The model under review builds one solid part; all positions refer to its coordinate system, in mm. Face numbers are marked on the shaded views. A direction names the side the tool comes from. Round coordinates to 2 decimals unless told otherwise and drop trailing zeros. Order: outer loops, then holes, each group sorted by start corner. A loop starts at its lowest first (then second) coordinate and runs counter-clockwise, first axis right, second up.
1) Machinability: for the marked faces 1 and 2, which of the approach directions +Z, -Z, +X, -X, +Y, -Y give a long, thin tool a straight path to every point of the face, cutting with its end or side? Answer none if there is none.
2) Consider section D-D (z = 58.5). Give the boundary of the cut face in (x, y).
3) Consider section A-A (z = 81.5). Give the boundary of the cut face in (x, y), then the cut area to 3 significant figures.
4) Clearance check with flat-ended pins moving along their axes: P1, Ø4, axis at x = -17.5, y = 30, coming from the -Z side; P2, Ø4, axis at x = -62, z = 31, coming from the +Y side; P3, Ø6, axis at x = 20, y = 43.5, coming from the +Z side; P4, Ø3, axis at x = 71, z = 31, coming from the -Y side. State where each tip first meets the part, or that it passes through.
5) To check wall thickness, follow L1, parallel to X at y = 2.5, z = 32; L2, parallel to Y at x = -85, z = 45.5; L3, parallel to X at y = -57.5, z = 76. State the ranges of each line that lie inside material, in increasing order.
6) Consider section C-C (y = 27.5). Give the boundary of the cut face in (x, z).
7) Consider section B-B (x = 53). Give the boundary of the cut face in (y, z), then the cut area to 3 significant figures.
from build123d import *
from build123d import SkipClean  # not in build123d's __all__

# Parameters (mm, degrees)
F1_DEPTH = 100
F3_DEPTH = 20
F4_DEPTH = 50


with BuildPart() as f1:
    # F0 (on Top) → F1 (new body)
    with BuildSketch(Plane.XY):
        with BuildLine():
            Line((-100, -50), (0, -50))
            Line((0, -50), (0, 0))
            Line((0, 0), (-75.3427499533, 0))
            ThreePointArc((-75.3427499533, 0), (-85.3427499533, -10), (-95.3427499533, 0))
            Line((-95.3427499533, 0), (-100, 0))
            Line((-100, 0), (-100, -50))
        make_face()
    extrude(amount=F1_DEPTH)

    # F2 (on face) → F3 (join)
    with BuildSketch(Plane.XZ.offset(50)):
        with BuildLine():
            ThreePointArc((0, 70), (-21.2132034356, 78.7867965644), (-30, 100))
            Line((-30, 100), (-60, 100))
            ThreePointArc((-60, 100), (-42.4264068712, 57.5735931288), (0, 40))
            Line((0, 40), (0, 70))
        make_face()
    extrude(amount=F3_DEPTH)

    # F4 (cut, through all): a face of the model
    f4_faces = [f1.faces().sort_by_distance(p)[0] for p in [
        (-12.7323954474, -50, 87.2676045526),
    ]]
    extrude(f4_faces, amount=-F4_DEPTH, mode=Mode.SUBTRACT)

    # F5: F1 across plane


with BuildPart() as f1_1:
    add(f1.part, clean=False)
    with SkipClean():  # cleaning this boolean's faces spoils the solid; the shape is the same uncleaned
        add(f1.part.mirror(Plane.XZ), clean=False)

    # F6: F1 across face


with BuildPart() as f1_2:
    add(f1_1.part, clean=False)
    add(f1_1.part.mirror(Plane(origin=(0, -30.1219512195, 37.9268292683), x_dir=(0, 1, 0), z_dir=(1, 0, 0))), clean=False)


solid = f1_2.part
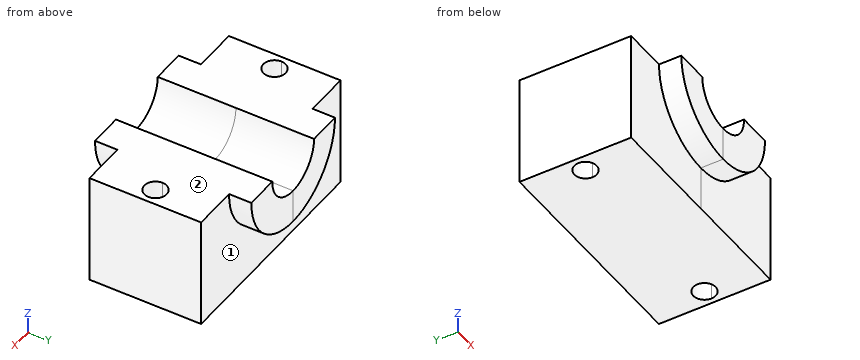
Answer below:
1. face 1: -Z, +Y
1. face 2: +Z, +X, -X, +Y, -Y
2. outline: (-100, -50) - (-43.33, -50) - (-43.33, -70) - (43.33, -70) - (43.33, -50) - (100, -50) - (100, 50) - (43.33, 50) - (43.33, 70) - (-43.33, 70) - (-43.33, 50) - (-100, 50) - close; hole circle Ø20 at (-85.34, 0); hole circle Ø20 at (85.34, 0)
3. outline: (-100, -50) - (-57.08, -50) - (-57.08, -70) - (-23.62, -70) - (-23.62, 70) - (-57.08, 70) - (-57.08, 50) - (-100, 50) - close; (23.62, -70) - (57.08, -70) - (57.08, -50) - (100, -50) - (100, 50) - (57.08, 50) - (57.08, 70) - (23.62, 70) - close; hole circle Ø20 at (-85.34, 0); hole circle Ø20 at (85.34, 0)
3. area: 17,300 mm2
4. P1: stops at z = 0
4. P2: stops at y = 50
4. P3: stops at z = 80.74
4. P4: stops at y = -50
5. L1: x = -100 to -95.03, -75.66 to 75.66, 95.03 to 100
5. L2: y = -50 to -9.99, 9.99 to 50
5. L3: x = -54.99 to -18, 18 to 54.99
6. outline: (-100, 0) - (100, 0) - (100, 100) - (30, 100) arc R30 cw to (-30, 100) - (-100, 100) - close
7. outline: (-70, 71.88) - (-50, 71.88) - (-50, 0) - (50, 0) - (50, 71.88) - (70, 71.88) - (70, 100) - (-70, 100) - close
7. area: 11,100 mm2
